Work out the finished part from the listing and answer in its coordinate system (mm). A direction names the side the tool comes from. Give positions to 0.01 mm unless a question says otherwise; leave off trailing zeros. Loops run counter-clockwise (first coordinate to the right, second up) from the corner with the lowest first, then second, coordinate; pieces in that order, holes last. Notation, with made-up numbers: (17, 46) -> (43, 46) arc R35 cw to (43, 80) -> close; hole circle Ø3 at (24, 35.25). An arc over 180 degrees is marked (long way). Answer as CSV lines item,"result". Start each with the question number.
1. Determine the mould class of faces 1 (the face through (-1, 1.35, -1)), 2 (the face through (-18, -2, 0)), 3 (the face through (-18, -1, -2)), 4 (the face through (-1, 1, 0)) for opening direction Z: +Z half, -Z half, draft (parallel to the pull), parting line (faces both ways), or undercut.
2. Find section A-A, the plane y = 3. Give the vertices of the cut face in (x, z) (3 decimals), and give its area (3 significant figures).
3. Find section D-D, the plane x = -24.5. Give the vertices of the cut face in (y, z), and give its area (3 significant figures).
4. Find section C-C, the plane y = -0.35. Give the vertices of the cut face in (x, z), and give its area (3 significant figures).
5. Find section B-B, the plane x = -6.5. Give the vertices of the cut face in (y, z).
6. Flat-ended cylindrical pins translate along their axes: pin 1 Ø1.6 at (x, z) = (0, 0) entering from +Y; pin 2 Ø1 at (y, z) = (2.5, 2.5) entering from -X; pin 3 Ø1.6 at (y, z) = (-1, 0.5) entering from +X. Find the tip coordinate at first contact, or state that the pin passes through.
7. A tool of negligible diameter and unlimited length cuts with its end or side. For faces 5 (the face through (-8.382, 0.666, 2.067)), 6 (the face through (-16, 1, 0)), 7 (the face through (-0.4, 0, 0)), 8 (the face through (-8.208, 0.666, -2.083)), from which of +Z, -Z, +X, -X, +Y, -Y can it reach the whole face along a straight path? Write none if from no direction.
8. Find the intervals of material crossed by line 1 along X through (y, z) = (1.8, 0) (3 decimals); line 2 along Z through (x, y) = (0, 0.85) (3 decimals); line 3 along X through (y, z) = (-1.35, -1.5), in increasing order.
from build123d import *

# Parameters (mm, degrees)
ESTRUSIONE_ESTRUSIONE1_DEPTH = 1.35
SCHIZZO2_R                   = 3.375
ESTRUSIONE_ESTRUSIONE2_DEPTH = 2
SCHIZZO3_R                   = 2.25
TAGLIO_ESTRUSIONE1_DEPTH     = 2
SCHIZZO4_R                   = 1
TAGLIO_ESTRUSIONE2_DEPTH     = 17.47393775
SCHIZZO6_W                   = 35
SCHIZZO6_H                   = 4
ESTRUSIONE_ESTRUSIONE3_DEPTH = 2


with BuildPart() as part:
    # Schizzo1 → Estrusione-Estrusione1 (new body)
    with BuildSketch(Plane(origin=(0, 0, 0), x_dir=(1, 0, 0), z_dir=(0, 1, 0))):
        with BuildLine():
            ThreePointArc((-2.090005981, -2.65), (-3.375, 0), (-2.090005981, 2.65))
            Line((-2.090005981, 2.65), (-14.5, 1.5))
            ThreePointArc((-14.5, 1.5), (-16, 0), (-14.5, -1.5))
            Line((-14.5, -1.5), (-2.090005981, -2.65))
        make_face()
        with BuildLine():
            ThreePointArc((3.375, 0), (1.472558117, 3.036807138), (-2.090005981, 2.65))
            Line((-2.090005981, 2.65), (-2.090005981, -2.65))
            ThreePointArc((-2.090005981, -2.65), (1.472558117, -3.036807138), (3.375, 0))
        make_face()
        with BuildLine():
            Line((-2.090005981, -2.65), (-2.090005981, 2.65))
            ThreePointArc((-2.090005981, 2.65), (-3.375, 0), (-2.090005981, -2.65))
        make_face()
    extrude(amount=ESTRUSIONE_ESTRUSIONE1_DEPTH)

    # Schizzo2 → Estrusione-Estrusione2 (add)
    with BuildSketch(Plane(origin=(0, 1.35, 0), x_dir=(1, 0, 0), z_dir=(0, 1, 0))):
        with Locations(Location((0, 0, 0), (0, 0, 128.262191128))):
            Circle(SCHIZZO2_R)
    extrude(amount=ESTRUSIONE_ESTRUSIONE2_DEPTH)

    # Schizzo3 → Taglio-Estrusione1 (cut)
    with BuildSketch(Plane(origin=(0, 3.35, 0), x_dir=(1, 0, 0), z_dir=(0, 1, 0))):
        with Locations(Location((0, 0, 0), (0, 0, 270))):
            Circle(SCHIZZO3_R)
    extrude(amount=-TAGLIO_ESTRUSIONE1_DEPTH, mode=Mode.SUBTRACT)

    # Schizzo4 → Taglio-Estrusione2 (cut, through all)
    with BuildSketch(Plane(origin=(0, 1.35, 0), x_dir=(1, 0, 0), z_dir=(0, 1, 0))):
        with Locations(Location((0, 0, 0), (0, 0, 270))):
            Circle(SCHIZZO4_R)
    extrude(amount=-TAGLIO_ESTRUSIONE2_DEPTH, mode=Mode.SUBTRACT)

    # Schizzo6 → Estrusione-Estrusione3 (add)
    with BuildSketch(Plane.XZ):
        with Locations((-17.5, 0)):
            Rectangle(SCHIZZO6_W, SCHIZZO6_H)
    extrude(amount=ESTRUSIONE_ESTRUSIONE3_DEPTH)


solid = part.part
Resolved:
1,face 1,"undercut"
1,face 2,"draft"
1,face 3,"-Z half"
1,face 4,"undercut"
2,outline,"circle Ø6.75 at (0, 0); hole circle Ø4.5 at (0, 0)"
2,area,"19.9 mm^2"
3,outline,"(-2, -2) -> (0, -2) -> (0, 2) -> (-2, 2) -> close"
3,area,"8.00 mm^2"
4,outline,"(-35, -2) -> (0, -2) -> (0, 2) -> (-35, 2) -> close"
4,area,"140 mm^2"
5,outline,"(-2, -2) -> (0, -2) -> (0, -2.24) -> (1.35, -2.24) -> (1.35, 2.24) -> (0, 2.24) -> (0, 2) -> (-2, 2) -> close"
6,pin 1,"stops at y = 0"
6,pin 2,"stops at x = -2.72"
6,pin 3,"stops at x = 0"
7,face 5,"+Z, -X, +Y"
7,face 6,"-X, +Y"
7,face 7,"+Y"
7,face 8,"-Z, -X, +Y"
8,line 1,"x = -3.375 to -2.25, 2.25 to 3.375"
8,line 2,"z = -3.375 to -1, 1 to 3.375"
8,line 3,"x = -35 to 0"
